Model file for the job. Use its own axes, mm. A direction names the side the tool comes from. Coordinates: 2 decimals unless noted, no trailing zeros. Loops run counter-clockwise (first coordinate to the right, second up) from the corner with the lowest first, then second, coordinate; pieces in that order, holes last.
from build123d import *

# Parameters (mm, degrees)
CYLINDER021_R     = 6
CYLINDER021_DEPTH = 6
CYLINDER020_R     = 2.1
CYLINDER020_DEPTH = 10


with BuildPart() as cylinder021:
    # Cylinder021 → Cylinder021 (new body)
    with BuildSketch(Plane.XY.offset(10)):
        Circle(CYLINDER021_R)
    extrude(amount=CYLINDER021_DEPTH)


with BuildPart() as fusion004:
    # Cylinder020 → Cylinder020 (new body)
    with BuildSketch(Plane.XY):
        Circle(CYLINDER020_R)
    extrude(amount=CYLINDER020_DEPTH)

    # Fusion004: union Cylinder021
    add(cylinder021.part)


with BuildPart() as fusion004_1:
    # Fusion004 placement: moved
    add(fusion004.part.moved(Location((-7, 12, -7))))


solid = fusion004_1.part
Q1. Drill centre lines: line 1 (Z direction, x = -9.25, y = 9.25); line 2 (X direction, y = 13.5, z = -1); line 3 (X direction, y = 11.75, z = 7.25). Where is each one in solid material? Low to high.
Answers:
line 1: z = 3 to 9
line 2: x = -8.47 to -5.53
line 3: x = -12.99 to -1.01
Q2. Slice it at A-A (y = 12). List the corners of the cut face in (x, z).
Answers:
outline: (-13, 3) - (-9.1, 3) - (-9.1, -7) - (-4.9, -7) - (-4.9, 3) - (-1, 3) - (-1, 9) - (-13, 9) - close
Q3. Which spindle directions (+Z, -Z, +X, -X, +Y, -Y) get a long thin tool onto all of the face, cutting with end or side? Do faces 1 (the flat face through (-7, 12, -7)), 2 (the cylindrical face through (-9.1, 12.09, -2.07)). Say none if no direction does.
Answers:
face 1: -Z, +X, -X, +Y, -Y
face 2: -Z
Q4. Slice it at B-B (x = -7). List the corners of the cut face in (y, z), and give its area (3 significant figures).
Answers:
outline: (6, 3) - (9.9, 3) - (9.9, -7) - (14.1, -7) - (14.1, 3) - (18, 3) - (18, 9) - (6, 9) - close
area: 114 mm2
Q5. Flat gauge pins, fed straight in: P1, Ø3, axis at y = 15.5, z = 5, coming from the +X side; P2, Ø3, axis at x = -11, z = 3, coming from the +Y side; P3, Ø5, axis at x = -9.5, z = -2, coming from the -Y side. Where does each tip first touch, or does it go through?
Answers:
P1: stops at x = -1.34
P2: stops at y = 17.45
P3: stops at y = 9.9
Q6. Slice it at D-D (z = 6.25). List the corners of the cut face in (x, y), and give its area (3 significant figures).
Answers:
outline: circle Ø12 at (-7, 12)
area: 113 mm2
Q7. Slice it at C-C (z = -3.5). List the corners of the cut face in (x, y).
Answers:
outline: circle Ø4.2 at (-7, 12)
